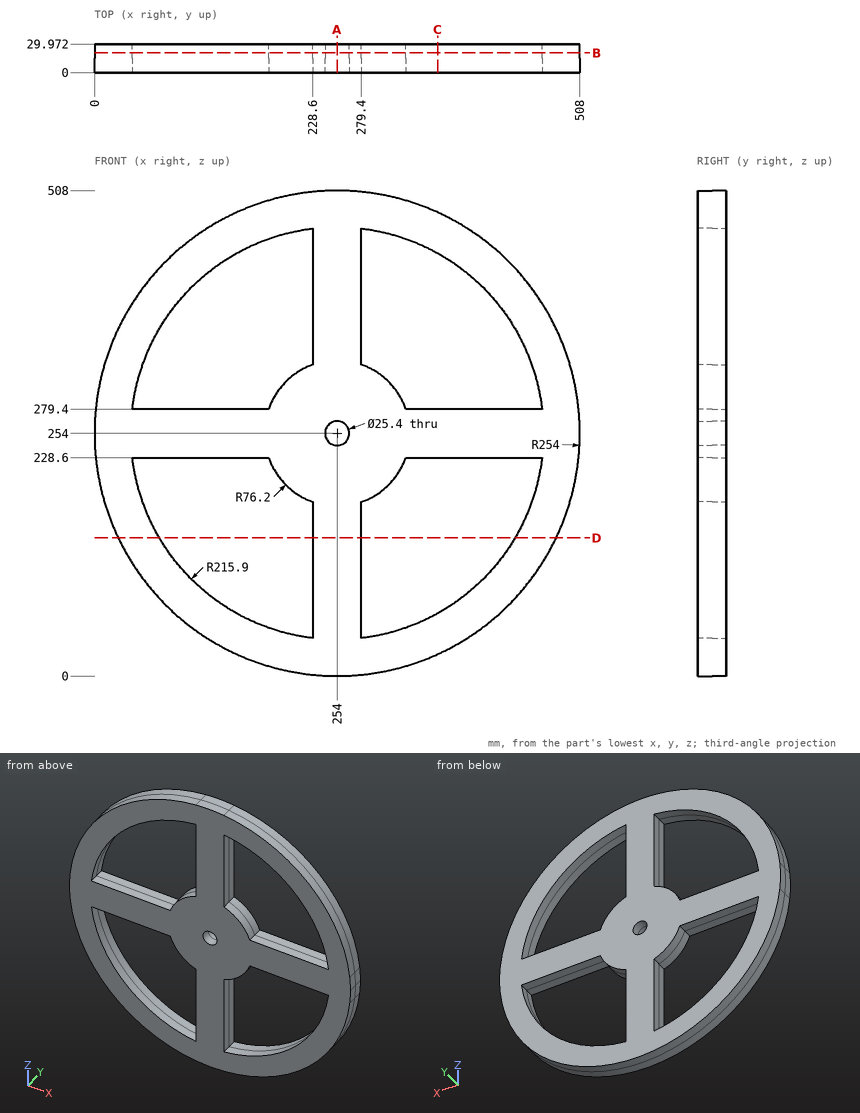
Source: three-view drawing plus pictorial views. Frame: mm from the lowest corner of the part. Round coordinates to 2 decimals unless told otherwise and drop trailing zeros. Loops run counter-clockwise (first coordinate to the right, second up) from the corner with the lowest first, then second, coordinate; pieces in that order, holes last. Notation, with made-up numbers: (30.25, -17.75) -> (77.25, -17.75) arc R15 ccw to (77.25, 1.25) -> close; hole circle Ø3 at (33, -39). An arc over 180 degrees is marked (long way). Use one line per item in the form item = value.
Item 1: Material intervals for probe 1 along Z at (x, y) = (254, 18.5); probe 2 along X at (y, z) = (11.25, 205); probe 3 along Z at (x, y) = (380, 4.5), sorted ascending.
Evaluation:
probe_1 = 0 to 241.3, 266.7 to 508
probe_2 = 4.77 to 43.73, 195.64 to 312.36, 464.27 to 503.23
probe_3 = 33.46 to 78.68, 228.6 to 279.4, 429.32 to 474.54
Item 2: Cut plane C-C on x = 359. Output: boundary loops of the cut face in (y, z).
Evaluation:
outline = (0, 22.72) -> (29.97, 22.72) -> (29.97, 65.35) -> (0, 65.35) -> close; (0, 228.6) -> (29.97, 228.6) -> (29.97, 279.4) -> (0, 279.4) -> close; (0, 442.65) -> (29.97, 442.65) -> (29.97, 485.28) -> (0, 485.28) -> close
Item 3: Cut plane B-B on y = 20.75. Output: boundary loops of the cut face in (x, z).
Evaluation:
outline = circle Ø508 at (254, 254); hole (39.6, 228.6) arc R215.9 ccw to (228.6, 39.6) -> (228.6, 182.16) arc R76.2 cw to (182.16, 228.6) -> close; hole (39.6, 279.4) -> (182.16, 279.4) arc R76.2 cw to (228.6, 325.84) -> (228.6, 468.4) arc R215.9 ccw to start; hole circle Ø25.4 at (254, 254); hole (279.4, 39.6) arc R215.9 ccw to (468.4, 228.6) -> (325.84, 228.6) arc R76.2 cw to (279.4, 182.16) -> close; hole (279.4, 325.84) arc R76.2 cw to (325.84, 279.4) -> (468.4, 279.4) arc R215.9 ccw to (279.4, 468.4) -> close
Item 4: Contact query for flat-ended pins moving along their axis: pin 1 Ø12 at (x, y) = (89.5, 7) entering from -Z; pin 2 Ø12 at (y, z) = (10.5, 362.5) entering from -X; pin 3 Ø7.5 at (y, z) = (10.5, 95.5) entering from +X. Output: stop coordinate, or through.
Evaluation:
pin_1 = 55.52
pin_2 = 21.6
pin_3 = 455.42
Item 5: Cut plane D-D on z = 144.5. Output: boundary loops of the cut face in (x, y), then the cut area to 3 significant figures.
Evaluation:
outline = (24.82, 0) -> (67.93, 0) -> (67.93, 29.97) -> (24.82, 29.97) -> close; (228.6, 0) -> (279.4, 0) -> (279.4, 29.97) -> (228.6, 29.97) -> close; (440.07, 0) -> (483.18, 0) -> (483.18, 29.97) -> (440.07, 29.97) -> close
area = 4,110 mm2
Item 6: Cut plane A-A on x = 254. Output: boundary loops of the cut face in (y, z), then the cut area to 3 significant figures.
Evaluation:
outline = (0, 0) -> (29.97, 0) -> (29.97, 241.3) -> (0, 241.3) -> close; (0, 266.7) -> (29.97, 266.7) -> (29.97, 508) -> (0, 508) -> close
area = 14,500 mm2
